Design review of the part built by this model. Coordinates are the model's own, in mm. A direction names the side the tool comes from. Coordinates: 2 decimals unless noted, no trailing zeros. Order: outer loops, then holes, each group sorted by start corner. A loop starts at its lowest first (then second) coordinate and runs counter-clockwise, first axis right, second up. Notation, with made-up numbers: (73.5, 24) - (80.5, 24) arc R14 cw to (80.5, 38) - close; hole circle Ø9 at (26.25, -7.75). An arc over 180 degrees is marked (long way). Write item = value, one per line. Start each with the question number.
```python
from build123d import *

# Parameters (mm, degrees)
F0_R          = 4.6355
F1_DEPTH      = 50.8
F2_D          = 8.4328
F2_DEPTH      = 38.1
F2_TIP        = 2.5334687141
F4_DEPTH      = 25.4
F4_DEPTH_BACK = 25.4
F5_ANGLE      = 90
F10_DEPTH     = 15.24


with BuildPart() as f1:
    # F0 (on Top) → F1 (new body)
    with BuildSketch(Plane.XY):
        Circle(F0_R)
    extrude(amount=F1_DEPTH)

    # F2
    with Locations(Plane(origin=(0, 0, 0), x_dir=(1, 0, 0), z_dir=(0, 0, -1))):
        with Locations((0, 0)):
            Hole(F2_D / 2, depth=F2_DEPTH)
            with Locations((0, 0, -(F2_DEPTH + F2_TIP / 2))):  # 118° drill point
                Cone(0, F2_D / 2, F2_TIP, mode=Mode.SUBTRACT)

    # F3 (on Front) → F4 (join, two sides)
    with BuildSketch(Plane.XZ) as f4_sk:
        Polygon((-9.627444493, 56.439600844), (-3.987843649, 50.8), (3.987756351, 50.8), (9.627357195, 56.439600844), (9.627357195, 64.415200844), (3.987756351, 70.0548016881), (-4.3649e-05, 70.0548016881), (-3.987843649, 70.0548016881), (-9.627444493, 64.415200844), align=None)
    extrude(amount=F4_DEPTH)
    extrude(f4_sk.sketch, amount=-F4_DEPTH_BACK)

    # F4_face (on face) → F5 (revolve)
    with BuildSketch(Plane(origin=(-4.3649e-05, -25.4, 60.427400844), x_dir=(1, 0, 0), z_dir=(0, -1, 0))):
        Polygon((9.627400844, 3.9878), (3.9878, 9.627400844), (-3.9878, 9.627400844), (-9.627400844, 3.9878), (-9.627400844, -3.9878), (-3.9878, -9.627400844), (3.9878, -9.627400844), (9.627400844, -3.9878), align=None)
    revolve(axis=Axis((-9.627444493, -25.4, 60.427400844), (0, 0, -1)), revolution_arc=F5_ANGLE)

    # F7 (on Right) → F8 (revolve)
    with BuildSketch(Plane.YZ):
        with BuildLine():
            ThreePointArc((30.9212189168, 51.2608121409), (37.4040035408, 53.9460694541), (40.089260854, 60.4288540781))
            ThreePointArc((40.089260854, 60.4288540781), (37.4040035408, 66.911638702), (30.9212189168, 69.5968960152))
            Line((30.9212189168, 69.5968960152), (30.9212189168, 60.4288540781))
            Line((30.9212189168, 60.4288540781), (30.9212189168, 51.2608121409))
        make_face()
    revolve(axis=Axis((0, 30.9212189168, 60.4288540781), (0, 0, -1)))

    # F9 (on face) → F10 (join)
    with BuildSketch(Plane(origin=(-9.627444493, 0, 0), x_dir=(0, -1, 0), z_dir=(-1, 0, 0))):
        Polygon((31.039600844, 50.8), (39.015200844, 50.8), (44.6548016881, 56.439600844), (44.6548016881, 64.415200844), (39.015200844, 70.0548016881), (31.039600844, 70.0548016881), (25.4, 64.415200844), (25.4, 56.439600844), align=None)
    extrude(amount=F10_DEPTH)


solid = f1.part
```
Item 1: Add section A-A on x = -13.5. Give the boundary of the cut face in (y, z), plus the area to 3 significant figures.
Item 2: Add section D-D on z = 12. Give the boundary of the cut face in (x, y).
Item 3: For faces 4 (the flat face through (-6.77, -0.36, 67.27)), 5 (the flat face through (6.3, 25.4, 56.3)), 6 (the cylindrical face through (-3.42, 3.13, 25.04)), 7 (the flat face through (-17.14, -28.18, 53.66)), list the 3-axis set-ups (+Z, -Z, +X, -X, +Y, -Y) from which the entire face can be reached by the end or side of a thin tool; tool diameter is ignored.
Item 4: Add section C-C on y = 15. Give the boundary of the cut face in (x, z).
Item 5: Mouldability with a two-part tool opening along Y and no side actions: class faces 1 (the cylindrical face through (0.55, -4.18, 19.32)), 2 (the flat face through (-17.14, -41.87, 67.2)), 3 (the flat face through (-9.627, 0, 60)) as +Y half, -Y half, draft (parallel to the pull), parting line (faces both ways), or undercut.
Item 6: For line 1 (Y direction, x = 0, z = 8); line 2 (Z direction, x = -2, y = -36); line 3 (Y direction, x = -2.5, z = 36.5), list the stretches that pass through material, from the lowest coordinate up.
Item 7: For P1, Ø9, axis at y = -6, z = 59, coming from the -X side; P2, Ø5, axis at y = -21, z = 52, coming from the -X side; P3, Ø2.5, axis at x = 0, y = 14, coming from the -Z side, all flat-tipped, find the tip position at first contact; note any pin that passes through.
Item 8: Add section B-B on z = 58. Give the boundary of the cut face in (x, y), plus the area to 3 significant figures.
Worked out:
q1.outline = (-44.65, 56.44) - (-39.02, 50.8) - (-31.04, 50.8) - (-25.4, 56.44) - (-25.4, 64.42) - (-31.04, 70.05) - (-39.02, 70.05) - (-44.65, 64.42) - close
q1.area = 307 mm2
q2.outline = circle Ø9.27 at (0, 0); hole circle Ø8.43 at (0, 0)
q3.face_4 = +Z, -X, +Y
q3.face_5 = none
q3.face_6 = -Z
q3.face_7 = -Z, -X, +Y
q4.outline = (-9.63, 56.44) - (-3.99, 50.8) - (3.99, 50.8) - (9.63, 56.44) - (9.63, 64.42) - (3.99, 70.05) - (-3.99, 70.05) - (-9.63, 64.42) - close
q5.face_1 = undercut
q5.face_2 = -Y half
q5.face_3 = draft
q6.line_1 = -4.64 to -4.22, 4.22 to 4.64
q6.line_2 = 50.8 to 70.05
q6.line_3 = -3.9 to -3.4, 3.4 to 3.9
q7.P1 = -9.63
q7.P2 = -7.69
q7.P3 = 50.8
q8.outline = (-24.87, -44.65) - (-9.63, -44.65) arc R19.25 ccw to (9.63, -25.4) - (9.63, 25.4) - (6.9, 25.4) arc R8.84 ccw (long way) to (-6.9, 25.4) - (-9.63, 25.4) - (-9.63, -25.4) - (-24.87, -25.4) - close
q8.area = 1,780 mm2
